Model file for the job. Use its own axes, mm. A direction names the side the tool comes from. Round coordinates to 2 decimals unless told otherwise and drop trailing zeros. Loops run counter-clockwise (first coordinate to the right, second up) from the corner with the lowest first, then second, coordinate; pieces in that order, holes last. Notation, with made-up numbers: (-13, 61) -> (42, 61) arc R17 cw to (42, 71) -> close; hole circle Ø7 at (36.25, -33.75). An arc over 180 degrees is marked (long way). Use a Markdown table: item, result.
from build123d import *

# Parameters (mm, degrees)
SKETCH_1_R      = 12
EXTRUDE_1_DEPTH = 23.5
SKETCH_2_R      = 1.5
EXTRUDE_2_DEPTH = 13.5
SKETCH_3_R      = 10.75
EXTRUDE_3_DEPTH = 5
SKETCH_4_R      = 4
EXTRUDE_4_DEPTH = 2
EXTRUDE_5_DEPTH = 2
EXTRUDE_6_DEPTH = 5


with BuildPart() as part:
    # 草图1 → 凸台-拉伸1 (new body)
    with BuildSketch(Plane(origin=(0, 0, 0), x_dir=(0, 0, -1), z_dir=(1, 0, 0))):
        Circle(SKETCH_1_R)
    extrude(amount=EXTRUDE_1_DEPTH)

    # 草图2 → 凸台-拉伸2 (add)
    with BuildSketch(Plane(origin=(23.5, 0, 0), x_dir=(0, 0, -1), z_dir=(1, 0, 0))):
        Circle(SKETCH_2_R)
    extrude(amount=EXTRUDE_2_DEPTH)

    # 草图3 → 凸台-拉伸3 (add)
    with BuildSketch(Plane(origin=(23.5, 0, 0), x_dir=(0, 0, -1), z_dir=(1, 0, 0))):
        Circle(SKETCH_3_R)
    extrude(amount=EXTRUDE_3_DEPTH)

    # 草图4 → 凸台-拉伸4 (add)
    with BuildSketch(Plane(origin=(28.5, 0, 0), x_dir=(0, 0, -1), z_dir=(1, 0, 0))):
        Circle(SKETCH_4_R)
    extrude(amount=EXTRUDE_4_DEPTH)

    # 草图5 → 凸台-拉伸5 (add)
    with BuildSketch(Plane.ZY):
        with BuildLine():
            Line((-2.061552813, -4), (2.061552813, -4))
            ThreePointArc((2.061552813, -4), (0, 4.5), (-2.061552813, -4))
        make_face()
    extrude(amount=EXTRUDE_5_DEPTH)

    # 草图6 → 凸台-拉伸6 (add)
    with BuildSketch(Plane.ZY):
        with BuildLine():
            Line((11.736694594, 2.5), (9, 2.5))
            Line((9, 2.5), (9, -2.5))
            Line((9, -2.5), (11.736694594, -2.5))
            ThreePointArc((11.736694594, -2.5), (11.933992105, -1.256913853), (12, 0))
            ThreePointArc((12, 0), (11.933992105, 1.256913853), (11.736694594, 2.5))
        make_face()
    extrude_6 = extrude(amount=EXTRUDE_6_DEPTH)

    # 镜向1: 凸台-拉伸6 across plane
    add(extrude_6.mirror(Plane.XY))


solid = part.part
Q1. Band-saw the part on D-D, the plane z = -2.5. Give the cut face in (x, y).
Results list:
| item | result |
|---|---|
| outline | (-2, -3.74) -> (0, -3.74) -> (0, -11.74) -> (23.5, -11.74) -> (23.5, -10.46) -> (28.5, -10.46) -> (28.5, -3.12) -> (30.5, -3.12) -> (30.5, 3.12) -> (28.5, 3.12) -> (28.5, 10.46) -> (23.5, 10.46) -> (23.5, 11.74) -> (0, 11.74) -> (0, 3.74) -> (-2, 3.74) -> close |
Q2. Flat gauge pins, fed straight in: pin 1 (3 mm diameter, centred on x = 22.5, z = 7.5, fed in from +Y); pin 2 (8 mm diameter, centred on x = 27, z = 9, fed in from -Y); pin 3 (12 mm diameter, centred on y = -3.5, z = -7, fed in from +X); pin 4 (12 mm diameter, centred on x = 23, z = -3.5, fed in from -Y). Where does each tip first touch, or does it go through?
Results list:
| item | result |
|---|---|
| pin 1 | stops at y = 10.39 |
| pin 2 | stops at y = -9.7 |
| pin 3 | stops at x = 30.5 |
| pin 4 | stops at y = -12 |
Q3. Tool access for faces 4 (the face through (-2, 2.5, -10)), 5 (the face through (-2, -2.5, 10)), 6 (the face through (-2, 0, 0)), 7 (the face through (-0.986, 4.497, 0.168)), 8 (the face through (23.5, -1, 11)): list every direction of +Z, -Z, +X, -X, +Y, -Y with a clear straight run to the whole face (end or side of a thin tool).
Results list:
| item | result |
|---|---|
| face 4 | -Z, -X, +Y |
| face 5 | +Z, -X, -Y |
| face 6 | -X, +Y, -Y |
| face 7 | -X |
| face 8 | +X |
Q4. Pull direction Z, two halves, no side cores. Call faces 1 (the face through (-2, 2.5, 10)), 2 (the face through (33.7, 0.07, 1.5)), 3 (the face through (-2, 0, 9)): released by +Z, released by -Z, zero draft, split by the parting line, or undercut.
Results list:
| item | result |
|---|---|
| face 1 | zero draft |
| face 2 | split by the parting line |
| face 3 | undercut |
Q5. Band-saw the part on A-A, the plane z = 0. Give the cut face in (x, y), plus the area to 3 significant figures.
Results list:
| item | result |
|---|---|
| outline | (-2, -4) -> (0, -4) -> (0, -12) -> (23.5, -12) -> (23.5, -10.75) -> (28.5, -10.75) -> (28.5, -4) -> (30.5, -4) -> (30.5, -1.5) -> (37, -1.5) -> (37, 1.5) -> (30.5, 1.5) -> (30.5, 4) -> (28.5, 4) -> (28.5, 10.75) -> (23.5, 10.75) -> (23.5, 12) -> (0, 12) -> (0, 4.5) -> (-2, 4.5) -> close |
| area | 724 mm² |
Q6. Drill centre lines: L1, parallel to X at y = -10.25, z = 4; L2, parallel to Z at x = 16.5, y = -0.5; L3, parallel to X at y = -6.25, z = 5.5. Where is each one in solid material? Low to high. Write a range as from..to.
Results list:
| item | result |
|---|---|
| L1 | x = 0..23.5 |
| L2 | z = -11.99..11.99 |
| L3 | x = 0..28.5 |
Q7. Band-saw the part on B-B, the plane y = 0.75. Give the cut face in (x, z).
Results list:
| item | result |
|---|---|
| outline | (-5, -11.98) -> (23.5, -11.98) -> (23.5, -10.72) -> (28.5, -10.72) -> (28.5, -3.93) -> (30.5, -3.93) -> (30.5, -1.3) -> (37, -1.3) -> (37, 1.3) -> (30.5, 1.3) -> (30.5, 3.93) -> (28.5, 3.93) -> (28.5, 10.72) -> (23.5, 10.72) -> (23.5, 11.98) -> (-5, 11.98) -> (-5, 9) -> (0, 9) -> (0, 4.44) -> (-2, 4.44) -> (-2, -4.44) -> (0, -4.44) -> (0, -9) -> (-5, -9) -> close |
Q8. Band-saw the part on C-C, the plane x = 7.5. Give the cut face in (y, z), plus the area to 3 significant figures.
Results list:
| item | result |
|---|---|
| outline | circle Ø24 at (0, 0) |
| area | 452 mm² |
